from build123d import *

# Parameters (mm, degrees)
BASE_FLANGE2_DEPTH           = 2
EDGE_FLANGE1_DEPTH           = 50
EDGE_FLANGE2_STRIP_W         = 13.2
EDGE_FLANGE2_STRIP_H         = 2
EDGE_FLANGE2_STRIP_CUT_DEPTH = 50
EDGE_FLANGE2_DEPTH           = 50
SKETCH18_R                   = 1.5
CUT_EXTRUDE1_DEPTH           = 10
EDGE_FLANGE3_STRIP_W         = 13.2
EDGE_FLANGE3_STRIP_H         = 2
EDGE_FLANGE3_STRIP_CUT_DEPTH = 50
EDGE_FLANGE3_DEPTH           = 50


# Sheet-metal steps are written as plain solids
with BuildPart() as part:
    # Sketch1 → Base-Flange2 (new body)
    with BuildSketch(Plane.XY):
        with BuildLine():
            Line((25.272889038, 31.228000671), (-24.727110962, 31.228000671))
            ThreePointArc((-24.727110962, 31.228000671), (-28.262644868, 29.763534577), (-29.727110962, 26.228000671))
            Line((-29.727110962, 26.228000671), (-29.727110962, -23.771999329))
            ThreePointArc((-29.727110962, -23.771999329), (-28.262644868, -27.307533234), (-24.727110962, -28.771999329))
            Line((-24.727110962, -28.771999329), (25.272889038, -28.771999329))
            ThreePointArc((25.272889038, -28.771999329), (28.808422944, -27.307533234), (30.272889038, -23.771999329))
            Line((30.272889038, -23.771999329), (30.272889038, 26.228000671))
            ThreePointArc((30.272889038, 26.228000671), (28.808422944, 29.763534577), (25.272889038, 31.228000671))
        make_face()
        with BuildLine():
            ThreePointArc((11.772817004, -4.771999329), (11.040605056, -3.004283311), (9.272889038, -2.272071362))
            ThreePointArc((9.272889038, -2.272071362), (7.505173021, -3.004283311), (6.772961072, -4.771999329))
            ThreePointArc((6.772961072, -4.771999329), (9.272889038, -7.271927295), (11.772817004, -4.771999329))
        make_face(mode=Mode.SUBTRACT)
        with BuildLine():
            ThreePointArc((-8.727110962, -2.272071362), (-10.494826979, -3.004283311), (-11.227038928, -4.771999329))
            ThreePointArc((-11.227038928, -4.771999329), (-8.727110962, -7.271927295), (-6.227182996, -4.771999329))
            ThreePointArc((-6.227182996, -4.771999329), (-6.959394944, -3.004283311), (-8.727110962, -2.272071362))
        make_face(mode=Mode.SUBTRACT)
        with BuildLine():
            ThreePointArc((6.772961072, 7.228000671), (9.272889038, 4.728072705), (11.772817004, 7.228000671))
            ThreePointArc((11.772817004, 7.228000671), (11.040605056, 8.995716689), (9.272889038, 9.727928638))
            ThreePointArc((9.272889038, 9.727928638), (7.505173021, 8.995716689), (6.772961072, 7.228000671))
        make_face(mode=Mode.SUBTRACT)
        with BuildLine():
            ThreePointArc((-8.727110962, 9.727928638), (-10.494826979, 8.995716689), (-11.227038928, 7.228000671))
            ThreePointArc((-11.227038928, 7.228000671), (-8.727110962, 4.728072705), (-6.227182996, 7.228000671))
            ThreePointArc((-6.227182996, 7.228000671), (-6.959394944, 8.995716689), (-8.727110962, 9.727928638))
        make_face(mode=Mode.SUBTRACT)
    extrude(amount=-BASE_FLANGE2_DEPTH)

    # Edge-Flange1 section (across the edge) → Edge-Flange1 (add)
    with BuildSketch(Plane(origin=(-24.727110962, 33.828000671, -2), x_dir=(0, -1, 0), z_dir=(1, 0, 0))):
        with BuildLine():
            Line((-2, 2.6), (-2, 43))
            Line((-2, 43), (0, 43))
            Line((0, 43), (0, 2.6))
            ThreePointArc((0, 2.6), (0.761522369, 0.761522369), (2.6, 0))
            Line((2.6, 0), (2.6, -2))
            ThreePointArc((2.6, -2), (-0.652691193, -0.652691193), (-2, 2.6))
        make_face()
    extrude(amount=EDGE_FLANGE1_DEPTH)

    # Edge-Flange2 strip (across the edge) → Edge-Flange2 strip cut (cut)
    with BuildSketch(Plane(origin=(25.272889038, 35.828000671, -45), x_dir=(0, 0, 1), z_dir=(-1, 0, 0))):
        with Locations((-2, -1)):
            Rectangle(EDGE_FLANGE2_STRIP_W, EDGE_FLANGE2_STRIP_H)
    extrude(amount=EDGE_FLANGE2_STRIP_CUT_DEPTH, mode=Mode.SUBTRACT)

    # Edge-Flange2 section (across the edge) → Edge-Flange2 (add)
    with BuildSketch(Plane(origin=(25.272889038, 35.828000671, -45), x_dir=(0, 0, 1), z_dir=(-1, 0, 0))):
        with BuildLine():
            Line((0, 2.6), (0, 13))
            Line((0, 13), (2, 13))
            Line((2, 13), (2, 2.6))
            ThreePointArc((2, 2.6), (2.761522369, 0.761522369), (4.6, 0))
            Line((4.6, 0), (4.6, -2))
            ThreePointArc((4.6, -2), (1.347308807, -0.652691193), (0, 2.6))
        make_face()
    extrude(amount=EDGE_FLANGE2_DEPTH)

    # Sketch18 → Cut-Extrude1 (cut)
    with BuildSketch(Plane(origin=(0, 0, -45), x_dir=(-1, 0, 0), z_dir=(0, 0, -1))):
        with Locations((-10, 43.828000671)):
            Circle(SKETCH18_R)
        with Locations((10, 43.828000671)):
            Circle(SKETCH18_R)
    extrude(amount=-CUT_EXTRUDE1_DEPTH, mode=Mode.SUBTRACT)

    # Edge-Flange3 strip (across the edge) → Edge-Flange3 strip cut (cut)
    with BuildSketch(Plane(origin=(-24.727110962, -28.771999329, 0), x_dir=(0, 1, 0), z_dir=(1, 0, 0))):
        with Locations((-2, -1)):
            Rectangle(EDGE_FLANGE3_STRIP_W, EDGE_FLANGE3_STRIP_H)
    extrude(amount=EDGE_FLANGE3_STRIP_CUT_DEPTH, mode=Mode.SUBTRACT)

    # Edge-Flange3 section (across the edge) → Edge-Flange3 (add)
    with BuildSketch(Plane(origin=(-24.727110962, -28.771999329, 0), x_dir=(0, 1, 0), z_dir=(1, 0, 0))):
        with BuildLine():
            Line((0, 2.6), (0, 18))
            Line((0, 18), (2, 18))
            Line((2, 18), (2, 2.6))
            ThreePointArc((2, 2.6), (2.761522369, 0.761522369), (4.6, 0))
            Line((4.6, 0), (4.6, -2))
            ThreePointArc((4.6, -2), (1.347308807, -0.652691193), (0, 2.6))
        make_face()
    extrude(amount=EDGE_FLANGE3_DEPTH)


solid = part.part
Model file for the job. Use its own axes, mm. A direction names the side the tool comes from. Coordinates: 2 decimals unless noted, no trailing zeros. Order: outer loops, then holes, each group sorted by start corner. A loop starts at its lowest first (then second) coordinate and runs counter-clockwise, first axis right, second up. Notation, with made-up numbers: (49.5, -18) -> (104.5, -18) arc R33 ccw to (104.5, 12) -> close; hole circle Ø6 at (8, -20). An arc over 180 degrees is marked (long way). Return JSON: item names as keys, results as strings. Group by question number.
Item 1: Tool access for faces 1 (the flat face through (0, 2, -2)), 2 (the flat face through (25.273, -28, -1)), 3 (the flat face through (25.273, -27, 9)): list every direction of +Z, -Z, +X, -X, +Y, -Y with a clear straight run to the whole face (end or side of a thin tool).
Item 2: Pull direction X, two halves, no side cores. Call faces 4 (the cylindrical face through (-0.08, -26.03, 0.78)), 5 (the cylindrical face through (28.85, 29.72, -0.99)), 6 (the cylindrical face through (-0.077, -27.389, -0.688)), 7 (the flat face through (-24.727, -27, 9)): pulls with the +X half, pulls with the -X half, needs draft (parallel to the pull), parting line crosses it, or undercut.
Item 3: Saw through at C-C on y = 0. Write the cut outline in (x, z), then the cut area to 3 significant figures.
Item 4: Saw through at B-B on z = -25. Write the cut outline in (x, y), then the cut area to 3 significant figures.
Item 5: Flat gauge pins, fed straight in: P1, Ø1, axis at y = -25.5, z = -1.5, coming from the +X side; P2, Ø19.5, axis at y = 44, z = -14, coming from the -X side; P3, Ø4, axis at x = 10, y = -5, coming from the +Z side; P4, Ø1.8, axis at x = -10, y = 43.828, coming from the -Z side. Where does each tip first touch, or does it go through?
Item 6: Wall check: line 1 along Z through (x, y) = (-13, -5.5); line 2 along Y through (x, z) = (-10, -5); line 3 along Y through (x, z) = (10, -44). Give the ranges that are in metal, low to high. Write a range as [from, to].
Item 7: Saw through at A-A on x = -14. Write the cut outline in (y, z), then the cut area to 3 significant figures.
Values found:
{
 "1": {"face 1": "-Z, +X, -X, -Y", "face 2": "-Z, -Y", "face 3": "+Z, +X, +Y, -Y"},
 "2": {"face 4": "needs draft", "face 5": "pulls with the +X half", "face 6": "undercut", "face 7": "pulls with the -X half"},
 "3": {"outline": "(-29.73, -2) -> (30.27, -2) -> (30.27, 0) -> (-29.73, 0) -> close", "area": "120 mm2"},
 "4": {"outline": "(-24.73, 33.83) -> (25.27, 33.83) -> (25.27, 35.83) -> (-24.73, 35.83) -> close", "area": "100 mm2"},
 "5": {"P1": "stops at x = 30.12", "P2": "stops at x = -24.73", "P3": "stops at z = 0", "P4": "passes through"},
 "6": {"line 1": "z = [-2, 0]", "line 2": "y = [33.83, 35.83]", "line 3": "y = [35.56, 42.33], [45.33, 48.83]"},
 "7": {"outline": "(-28.77, 2.6) arc R4.6 ccw to (-24.17, -2) -> (31.23, -2) arc R2.6 cw to (33.83, -4.6) -> (33.83, -40.4) arc R4.6 ccw to (38.43, -45) -> (48.83, -45) -> (48.83, -43) -> (38.43, -43) arc R2.6 cw to (35.83, -40.4) -> (35.83, -4.6) arc R4.6 ccw to (31.23, 0) -> (-24.17, 0) arc R2.6 cw to (-26.77, 2.6) -> (-26.77, 18) -> (-28.77, 18) -> close", "area": "268 mm2"}
}
